Model file for the job. Use its own axes, mm. Face numbers are marked on the shaded views. A direction names the side the tool comes from. Round coordinates to 2 decimals unless told otherwise and drop trailing zeros. Loops run counter-clockwise (first coordinate to the right, second up) from the corner with the lowest first, then second, coordinate; pieces in that order, holes last. Notation, with made-up numbers: (79.5, 24) -> (130.5, 24) arc R15 cw to (130.5, 49) -> close; hole circle Ø8 at (54, -23.75). An arc over 180 degrees is marked (long way). Use a Markdown table: item, result.
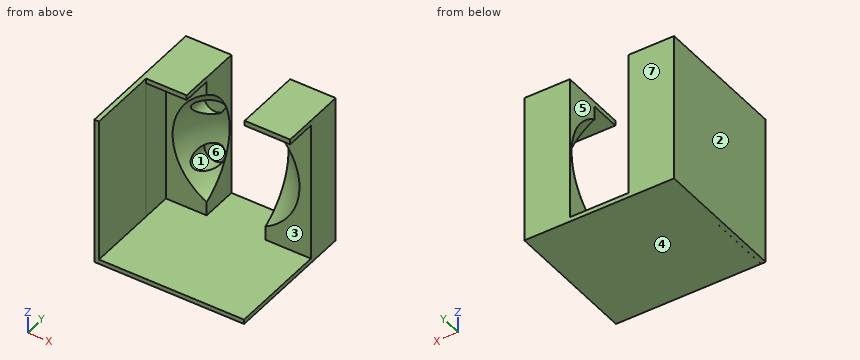
from build123d import *
from build123d.topology import SkipClean

# Parameters (mm, degrees)
SKETCH1_W                   = 102
SKETCH1_H                   = 102
BOSS_EXTRUDE1_DEPTH         = 50
CUT_EXTRUDE_THIN1_OUTLINE_W = 40
CUT_EXTRUDE_THIN1_OUTLINE_H = 95.773670058
CUT_EXTRUDE_THIN1_DEPTH     = 50
SKETCH4_W                   = 40
SKETCH4_H                   = 6.202657501
CUT_EXTRUDE3_DEPTH          = 54
SKETCH5_W                   = 33.817621941
SKETCH5_H                   = 102.594578927
CUT_EXTRUDE4_DEPTH          = 20
SKETCH6_W                   = 27.820383201
SKETCH6_H                   = 98.886835029
CUT_EXTRUDE5_DEPTH          = 20
SKETCH7_W                   = 30.8
SKETCH7_H                   = 3.364819678
BOSS_EXTRUDE2_DEPTH         = 21
SKETCH9_W                   = 31
SKETCH9_H                   = 3.479961613
BOSS_EXTRUDE4_DEPTH         = 21
SKETCH10_W                  = 3.15002448
SKETCH10_H                  = 102
BOSS_EXTRUDE5_DEPTH         = 47.625
SKETCH11_W                  = 98.820383201
SKETCH11_H                  = 3.113164971
BOSS_EXTRUDE6_DEPTH         = 47.625
SKETCH14_W                  = 102
SKETCH14_H                  = 5
CUT_EXTRUDE7_DEPTH          = 105
SKETCH13_R                  = 7.5
CUT_EXTRUDE8_DEPTH          = 20
SKETCH13_4_R                = 7.5
CUT_EXTRUDE9_DEPTH          = 20


# Read off the part's stored shape, not the designer's step: Cut-Extrude-Thin1
with BuildPart() as part:
    # Sketch1 → Boss-Extrude1 (new body)
    with BuildSketch(Plane(origin=(0, 0, 0), x_dir=(1, 0, 0), z_dir=(0, 1, 0))):
        with Locations((-66.567363259, 25.977216604)):
            Rectangle(SKETCH1_W, SKETCH1_H)
    extrude(amount=BOSS_EXTRUDE1_DEPTH)

    # Sketch2 → Cut-Revolve1 (revolve, cut)
    with SkipClean():  # the faces are left unmerged after this step: merging them gives an invalid solid
        with BuildSketch(Plane(origin=(0, 0, 0), x_dir=(1, 0, 0), z_dir=(0, 1, 0))):
            with BuildLine():
                ThreePointArc((-66.567363259, 73.602216604), (-114.192363259, 25.977216604), (-66.567363259, -21.647783396))
                Line((-66.567363259, -21.647783396), (-66.567363259, 73.602216604))
            make_face()
            with BuildLine():
                Line((-66.567363259, 73.602216604), (-66.567363259, -21.647783396))
                ThreePointArc((-66.567363259, -21.647783396), (-32.891402805, -7.69874385), (-18.942363259, 25.977216604))
                ThreePointArc((-18.942363259, 25.977216604), (-32.891402805, 59.653177058), (-66.567363259, 73.602216604))
            make_face()
        revolve(axis=Axis((-66.567363259, 0, 21.647783396), (0, 0, -1)), mode=Mode.SUBTRACT)
    add(part.part.scale(1), mode=Mode.REPLACE)  # the faces are merged on a copy

    # Cut-Extrude-Thin1 outline → Cut-Extrude-Thin1 (cut)
    with BuildSketch(Plane(origin=(0, 0, 0), x_dir=(1, 0, 0), z_dir=(0, 1, 0))):
        with Locations((-66.567363259, 25.977216604)):
            Rectangle(CUT_EXTRUDE_THIN1_OUTLINE_W, CUT_EXTRUDE_THIN1_OUTLINE_H)
    extrude(amount=CUT_EXTRUDE_THIN1_DEPTH, mode=Mode.SUBTRACT)

    # Sketch4 → Cut-Extrude3 (cut)
    with BuildSketch(Plane(origin=(0, 0, 0), x_dir=(1, 0, 0), z_dir=(0, 1, 0))):
        with Locations((-66.567363259, -25.010947176)):
            Rectangle(SKETCH4_W, SKETCH4_H)
    extrude(amount=CUT_EXTRUDE3_DEPTH, mode=Mode.SUBTRACT)

    # Sketch5 → Cut-Extrude4 (cut)
    with BuildSketch(Plane(origin=(0, 0, 0), x_dir=(1, 0, 0), z_dir=(0, 1, 0))):
        with Locations((-29.658552289, 22.56676217)):
            Rectangle(SKETCH5_W, SKETCH5_H)
    extrude(amount=CUT_EXTRUDE4_DEPTH, mode=Mode.SUBTRACT)

    # Sketch6 → Cut-Extrude5 (cut)
    with BuildSketch(Plane(origin=(0, 0, 0), x_dir=(-1, 0, 0), z_dir=(0, -1, 0))):
        with Locations((100.47755486, 24.420634119)):
            Rectangle(SKETCH6_W, SKETCH6_H)
    extrude(amount=-CUT_EXTRUDE5_DEPTH, mode=Mode.SUBTRACT)

    # Sketch7 → Boss-Extrude2 (add)
    with BuildSketch(Plane(origin=(0, 0, 0), x_dir=(1, 0, 0), z_dir=(0, 1, 0))):
        with Locations((-102.167363259, -23.340373557)):
            Rectangle(SKETCH7_W, SKETCH7_H)
    extrude(amount=BOSS_EXTRUDE2_DEPTH)

    # Sketch9 → Boss-Extrude4 (add)
    with BuildSketch(Plane.XZ.offset(-20)):
        with Locations((-31.067363259, 23.28280259)):
            Rectangle(SKETCH9_W, SKETCH9_H)
    extrude(amount=BOSS_EXTRUDE4_DEPTH)

    # Sketch10 → Boss-Extrude5 (add)
    with BuildSketch(Plane.XZ):
        with Locations((-115.992351019, -25.977216604)):
            Rectangle(SKETCH10_W, SKETCH10_H)
    extrude(amount=BOSS_EXTRUDE5_DEPTH)

    # Sketch11 → Boss-Extrude6 (add)
    with BuildSketch(Plane.XZ):
        with Locations((-64.97755486, -75.420634119)):
            Rectangle(SKETCH11_W, SKETCH11_H)
    extrude(amount=BOSS_EXTRUDE6_DEPTH)

    # Sketch14 → Cut-Extrude7 (cut)
    with BuildSketch(Plane(origin=(-15.567363259, 0, 0), x_dir=(0, 0, -1), z_dir=(1, 0, 0))):
        with Locations((25.977216604, 47.5)):
            Rectangle(SKETCH14_W, SKETCH14_H)
    extrude(amount=-CUT_EXTRUDE7_DEPTH, mode=Mode.SUBTRACT)

    # Sketch13 → Cut-Extrude8 (cut)
    with BuildSketch(Plane.XZ.offset(-20)):
        with Locations((-94.167363259, -8.342036282)):
            Circle(SKETCH13_R)
    extrude(amount=-CUT_EXTRUDE8_DEPTH, mode=Mode.SUBTRACT)

    # Sketch13<4> → Cut-Extrude9 (cut)
    with BuildSketch(Plane.XZ.offset(-20)):
        with Locations((-94.167363259, -43.864051633)):
            Circle(SKETCH13_4_R)
    extrude(amount=-CUT_EXTRUDE9_DEPTH, mode=Mode.SUBTRACT)


solid = part.part
Q1. Band-saw the part on C-C, the plane y = 14. Give the cut face in (x, z).
Results list:
| item | result |
|---|---|
| outline | (-117.57, -76.98) -> (-15.57, -76.98) -> (-15.57, -73.86) -> (-114.39, -73.86) -> (-114.39, 21.66) -> (-86.77, 21.66) -> (-86.77, 25.02) -> (-117.57, 25.02) -> close; (-46.57, 21.54) -> (-15.57, 21.54) -> (-15.57, 25.02) -> (-46.57, 25.02) -> close |
Q2. Flat gauge pins, fed straight in: pin 1 (9 mm diameter, centred on x = -94.17, z = -43.86, fed in from -Y); pin 2 (4 mm diameter, centred on x = -39.5, y = -21.5, fed in from +Z); pin 3 (8.5 mm diameter, centred on x = -95, z = -24, fed in from -Y). Where does each tip first touch, or does it go through?
Results list:
| item | result |
|---|---|
| pin 1 | stops at y = 40 |
| pin 2 | stops at z = -73.86 |
| pin 3 | stops at y = 34.58 |
Q3. Tool access for the marked faces 5, 6 and 7: list every direction of +Z, -Z, +X, -X, +Y, -Y with a clear straight run to the whole face (end or side of a thin tool).
Results list:
| item | result |
|---|---|
| face 5 | +Z, +Y, -Y |
| face 6 | -Y |
| face 7 | +Z, -Z, +X, -X, +Y |
Q4. Pull direction Z, two halves, no side cores. Call the marked faces 1, 2, 3 and 4: released by +Z, released by -Z, zero draft, split by the parting line, or undercut.
Results list:
| item | result |
|---|---|
| face 1 | undercut |
| face 2 | zero draft |
| face 3 | undercut |
| face 4 | released by -Z |
Q5. Band-saw the part on A-A, the plane z = 15. Give the cut face in (x, y) (3 decimals), plus the area to 3 significant figures.
Results list:
| item | result |
|---|---|
| outline | (-117.567, -47.625) -> (-114.417, -47.625) -> (-114.417, 0) -> (-114.388, 0) -> (-114.388, 20) -> (-86.567, 20) -> (-86.567, 45) -> (-117.567, 45) -> close; (-46.567, 20) -> (-15.567, 20) -> (-15.567, 45) -> (-46.567, 45) -> close |
| area | 1,760 mm² |
Q6. Band-saw the part on B-B, the plane y = -37. Give the cut face in (x, z), plus the area to 3 significant figures.
Results list:
| item | result |
|---|---|
| outline | (-117.57, -76.98) -> (-114.42, -76.98) -> (-114.42, 25.02) -> (-117.57, 25.02) -> close; (-114.39, -76.98) -> (-15.57, -76.98) -> (-15.57, -73.86) -> (-114.39, -73.86) -> close |
| area | 629 mm² |
Q7. Drill centre lines: L1, parallel to X at y = 24, z = -69; L2, parallel to Z at x = -61, y = 9; L3, parallel to Y at x = -21, z = -65. Where is each one in solid material? Low to high. Write a range as from..to.
Results list:
| item | result |
|---|---|
| L1 | x = -117.57..-86.57, -46.57..-15.57 |
| L2 | z = -76.98..-73.86 |
| L3 | y = 20..45 |
Q8. Band-saw the part on D-D, the plane x = -33.5. Give the cut face in (y, z) (1 decimal), plus the area to 3 significant figures.
Results list:
| item | result |
|---|---|
| outline | (-47.6, -77) -> (45, -77) -> (45, 25) -> (-1, 25) -> (-1, 21.5) -> (20, 21.5) -> (20, 1.9) arc R34.3 cw to (20, -53.8) -> (20, -73.9) -> (-47.6, -73.9) -> close |
| area | 2,280 mm² |
